Read the model definition and answer for the solid it produces. Units are mm, in the model's axes. A direction names the side the tool comes from. Coordinates: 2 decimals unless noted, no trailing zeros. Write each loop counter-clockwise with the first axis right and the second up, starting at its lowest first coordinate (ties: lowest second). Pieces come first, ordered by that corner, then holes. Notation, with made-up numbers: (72, -34) -> (78, -34) arc R16 ccw to (78, -12) -> close; hole circle Ø5 at (14.25, 37). An arc over 180 degrees is marked (long way). Use CSV: the item, a comma, the result in double quotes. Start each with the question number.
from build123d import *

# Parameters (mm, degrees)
CUT_EXTRUDE1_DEPTH           = 3
CIRPATTERN1_COUNT            = 3
M10_TAPPED_HOLE1_D           = 8.5
M10_TAPPED_HOLE1_DEPTH       = 24.5
M10_TAPPED_HOLE1_CBORE_D     = 10
M10_TAPPED_HOLE1_CBORE_DEPTH = 20
M10_TAPPED_HOLE1_TIP         = 2.553657631


with BuildPart() as part:
    # Sketch1 → Revolve1 (revolve)
    with BuildSketch(Plane.XY, mode=Mode.PRIVATE) as revolve1_sk:
        Polygon((0, 13.5), (0, 17.5), (50, 30), (91, 30), (91, 24), (99, 24), (99, 30), (104, 30), (110, 26.535898385), (110, 0), (17.216878365, 0), (10, 12.5), (1, 12.5), align=None)
    revolve(revolve1_sk.sketch.rotate(Axis((0, 0, 0), (1, 0, 0)), 90), axis=Axis((0, 0, 0), (1, 0, 0)))

    # Sketch2 → Cut-Extrude1 (cut, symmetric)
    with BuildSketch(Plane.XY):
        with BuildLine():
            Line((98, 13), (110, 13))
            Line((110, 13), (110, 30))
            Line((110, 30), (60.436720058, 30))
            ThreePointArc((60.436720058, 30), (77.384471872, 17.447832104), (98, 13))
        make_face()
    cut_extrude1 = extrude(amount=CUT_EXTRUDE1_DEPTH, both=True, mode=Mode.SUBTRACT)

    # CirPattern1: Cut-Extrude1 ×3 about axis
    cirpattern1_axis = Axis((0, 0, 0), (1, 0, 0))
    for i in range(1, CIRPATTERN1_COUNT):
        add(cut_extrude1.rotate(cirpattern1_axis, i * 360 / CIRPATTERN1_COUNT), mode=Mode.SUBTRACT)

    # M10 Tapped Hole1
    with Locations(Plane(origin=(110, 0, 0), x_dir=(0, 0, -1), z_dir=(1, 0, 0))):
        with Locations((0, 0)):
            CounterBoreHole(M10_TAPPED_HOLE1_D / 2, M10_TAPPED_HOLE1_CBORE_D / 2, M10_TAPPED_HOLE1_CBORE_DEPTH, depth=M10_TAPPED_HOLE1_DEPTH)
            with Locations((0, 0, -(M10_TAPPED_HOLE1_DEPTH + M10_TAPPED_HOLE1_TIP / 2))):  # 118° drill point
                Cone(0, M10_TAPPED_HOLE1_D / 2, M10_TAPPED_HOLE1_TIP, mode=Mode.SUBTRACT)


solid = part.part
1) Each of these flat-tipped pins is pushed along its axis until it touches: pin 1 (13.5 mm diameter, centred on x = 80.5, y = 19.5, fed in from +Z); pin 2 (9 mm diameter, centred on y = 0, z = 0, fed in from -X); pin 3 (5 mm diameter, centred on x = 74, y = 20, fed in from -Z). Where does it stop, or does it pass through?
2) The mould has two halves that part along X. Classify faces 1 (the face through (91, 12, -22)), 2 (the face through (0, 10.3, -9)), 3 (the face through (95.06, 11.73, -20.94)), 4 (the face through (110, 5.4, -0.4)): pulls with the +X half, pulls with the -X half, needs draft (parallel to the pull), parting line crosses it, or undercut.
3) Section B-B, the plane x = 24 is taken. Give the vertices of the cut face in (y, z).
4) Find the intervals of material crossed by line 1 along Z through (x, y) = (96.5, -5.5); line 2 along Y through (x, z) = (97, 0); line 3 along Y through (x, z) = (105.5, -19), in increasing order.
5) Which of the six approach directions +Z, -Z, +X, -X, +Y, -Y give full straight-line access (tool end or side, diameter ignored) to faces 5 (the face through (87.718, 3.584, 2.285)), 6 (the face through (77.114, 17.571, 0.042)), 7 (the face through (95, -24, 0))?
6) Section A-A, the plane x = 66.5 is taken. Give the vertices of the cut face in (y, z).
The answers:
1,pin 1,"stops at z = 27.16"
1,pin 2,"stops at x = 14.62"
1,pin 3,"stops at z = -24.37"
2,face 1,"undercut"
2,face 2,"pulls with the -X half"
2,face 3,"undercut"
2,face 4,"pulls with the +X half"
3,outline,"circle Ø47 at (0, 0)"
4,line 1,"z = -23.36 to -15.53, -11.86 to 11.86, 15.53 to 23.36"
4,line 2,"y = -24 to -5, 5 to 13.01"
4,line 3,"y = -22.09 to -14.43, -7.51 to 22.09"
5,face 5,"+X"
5,face 6,"+X, +Y"
5,face 7,"-Y"
6,outline,"(-17.52, -24.35) -> (-14.68, -19.43) -> (-9.49, -22.43) -> (-12.33, -27.35) arc R30 ccw to (29.85, -3) -> (24.17, -3) -> (24.17, 3) -> (29.85, 3) arc R30 ccw to (-12.33, 27.35) -> (-9.49, 22.43) -> (-14.68, 19.43) -> (-17.52, 24.35) arc R30 ccw to start"
